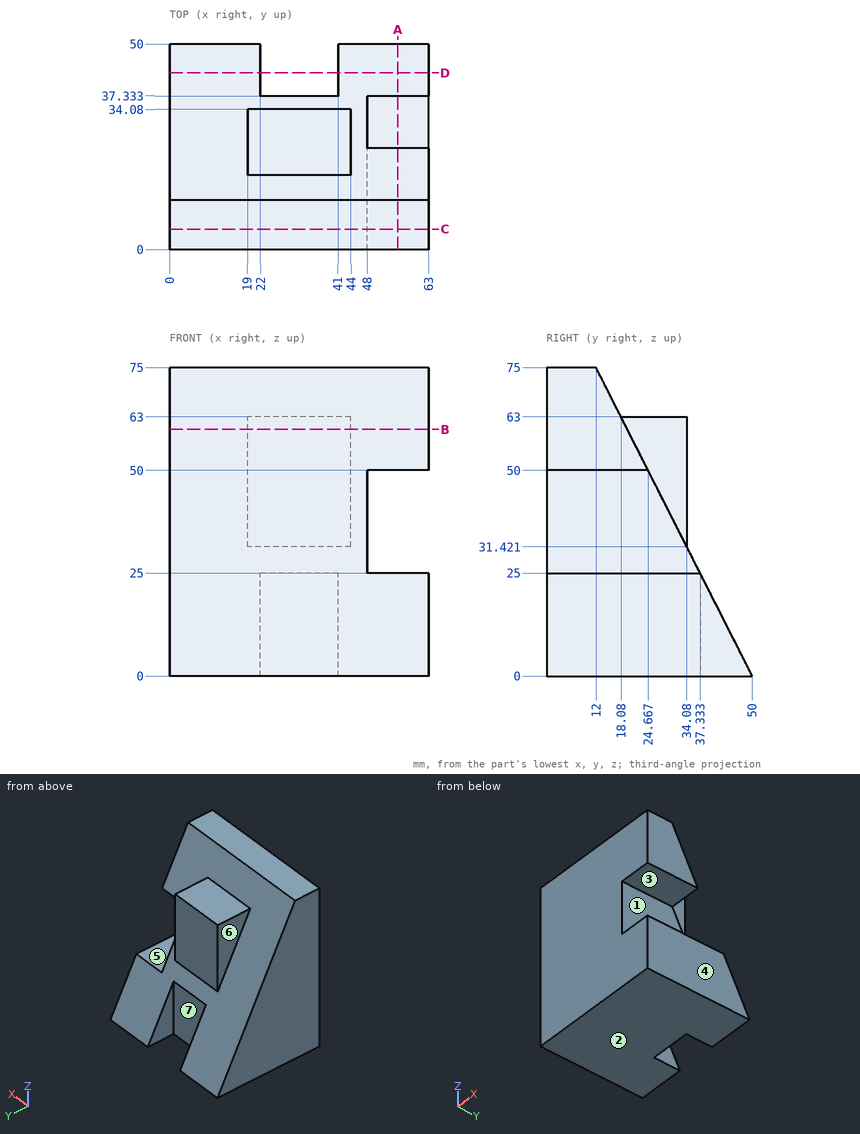
Study the drawing (mm; zero at the part's minimum x, y, z) and answer. A direction names the side the tool comes from. Coordinates: 2 decimals unless noted, no trailing zeros. Write each loop counter-clockwise with the first axis right and the second up, starting at its lowest first coordinate (ties: lowest second). Pieces come first, ordered by that corner, then holes. Notation, with made-up numbers: (57.5, -38.5) - (73.5, -38.5) arc R13 cw to (73.5, -16.5) - close; hole circle Ø5 at (77, 44.5). An arc over 180 degrees is marked (long way). Answer as a JSON object with one key per item and string values.
Q1. For a pull along Z with two mould halves and no side action, classify the marked faces 1, 2, 3 and 4 as pulls with the +Z half, pulls with the -Z half, needs draft (parallel to the pull), parting line crosses it, or undercut.
Results list:
{"face 1": "undercut", "face 2": "pulls with the -Z half", "face 3": "undercut", "face 4": "needs draft"}
Q2. Consider L1, parallel to X at y = 39, z = 7.5; L2, parallel to Y at x = 30, z = 44; L3, parallel to Y at x = 33, z = 4. Determine where each line is inside the solid, lowest interval first. Write a range as from..to.
Results list:
{"L1": "x = 0..22, 41..63", "L2": "y = 0..34.08", "L3": "y = 0..37.33"}
Q3. Find section B-B (z = 60). Write down the section's boundary in (x, y).
Results list:
{"outline": "(0, 0) - (63, 0) - (63, 19.6) - (44, 19.6) - (44, 34.08) - (19, 34.08) - (19, 19.6) - (0, 19.6) - close"}
Q4. Find section C-C (y = 5). Write down the section's boundary in (x, z), plus the area to 3 significant figures.
Results list:
{"outline": "(0, 0) - (63, 0) - (63, 25) - (48, 25) - (48, 50) - (63, 50) - (63, 75) - (0, 75) - close", "area": "4,350 mm^2"}
Q5. Given pin 1 Ø8 at (y, z) = (29.5, 48.5) entering from +X; pin 2 Ø10 at (x, y) = (10.5, 16.5) entering from +Z; pin 3 Ø1.5 at (x, z) = (10.5, 49) entering from +Y; pin 4 Ø5.5 at (x, z) = (28, 18.5) entering from +Y, each flat-ended and moving along its own axis, determine where each tip first touches the part or whether it passes through.
Results list:
{"pin 1": "stops at x = 48", "pin 2": "stops at z = 75", "pin 3": "stops at y = 25.55", "pin 4": "stops at y = 37.33"}
Q6. Which of the six approach directions +Z, -Z, +X, -X, +Y, -Y give full straight-line access (tool end or side, diameter ignored) to the marked faces 5, 6 and 7?
Results list:
{"face 5": "+X, +Y, -Y", "face 6": "+Z, -X, +Y", "face 7": "+Z, -Z, +Y"}
Q7. Find section A-A (x = 55.5). Write down the section's boundary in (y, z).
Results list:
{"outline": "(0, 0) - (50, 0) - (37.33, 25) - (0, 25) - close; (0, 50) - (24.67, 50) - (12, 75) - (0, 75) - close"}
Q8. Find section D-D (y = 43). Write down the section's boundary in (x, z).
Results list:
{"outline": "(0, 0) - (22, 0) - (22, 13.82) - (0, 13.82) - close; (41, 0) - (63, 0) - (63, 13.82) - (41, 13.82) - close"}
